Could you check a few things on this drawing? It's one solid part, dimensions in mm from its lowest x, y, z. A direction names the side the tool comes from. Give positions to 0.01 mm unless a question says otherwise; leave off trailing zeros. Order: outer loops, then holes, each group sorted by start corner. A loop starts at its lowest first (then second) coordinate and runs counter-clockwise, first axis right, second up. Notation, with made-up numbers: M -28.75,8 L -7.75,8 A19 cw -7.75,27 Z; hole C 53,3 d4. An arc over 180 degrees is marked long. Use one line per item in the form item = value.
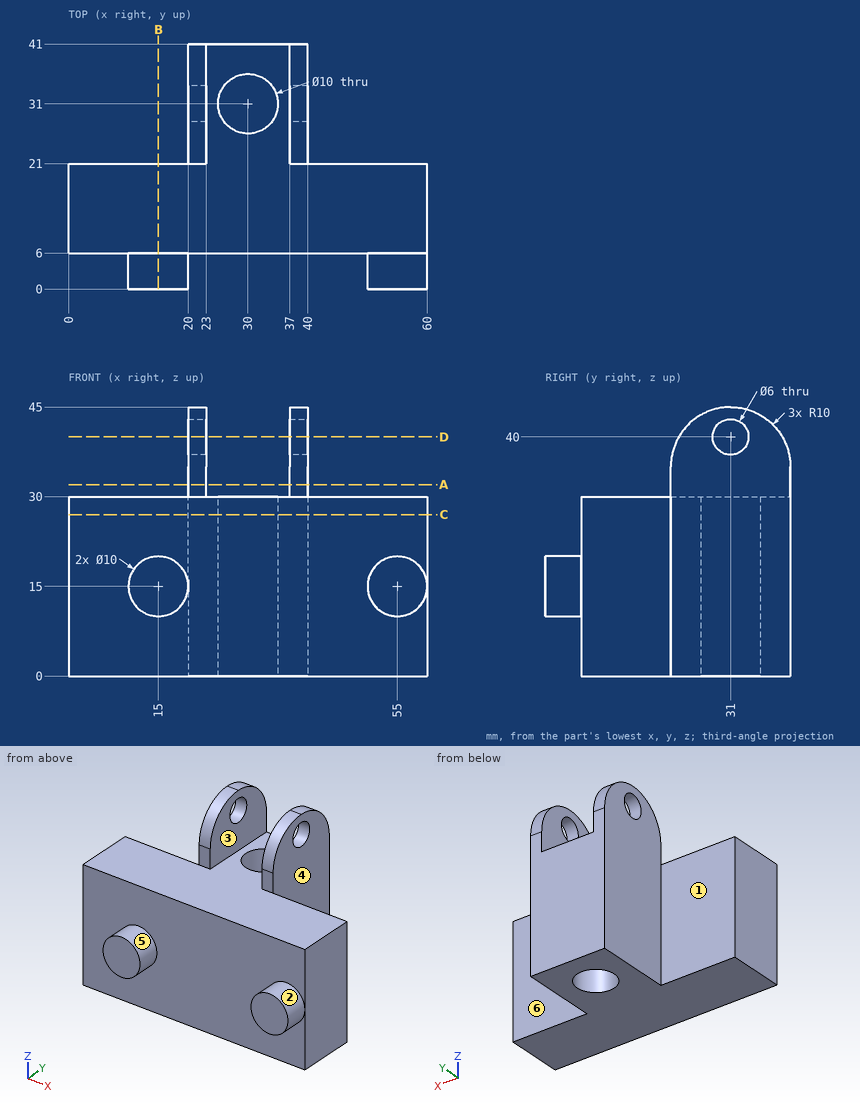
Q1. I want a section at D-D on z = 40. Write out the boundary of the cut face in (x, y), then the cut area to 3 significant figures.
Found:
outline = M 20,22.34 L 23,22.34 L 23,28 L 20,28 Z; M 20,34 L 23,34 L 23,39.66 L 20,39.66 Z; M 37,22.34 L 40,22.34 L 40,28 L 37,28 Z; M 37,34 L 40,34 L 40,39.66 L 37,39.66 Z
area = 67.9 mm²
Q2. I want a section at A-A on z = 32. Write out the boundary of the cut face in (x, y).
Found:
outline = M 20,21 L 23,21 L 23,41 L 20,41 Z; M 37,21 L 40,21 L 40,41 L 37,41 Z
Q3. I want a section at C-C on z = 27. Write out the boundary of the cut face in (x, y).
Found:
outline = M 0,6 L 60,6 L 60,21 L 40,21 L 40,41 L 20,41 L 20,21 L 0,21 Z; hole C 30,31 d10
Q4. I need wall thicknesses on L1, parallel to X at y = 27, z = 36; L2, parallel to X at y = 39, z = 4; L3, parallel to Z at x = 51, y = 8.5. Which ranges of each line are inside material? Lowest first, please.
Found:
L1 = 20 to 23, 37 to 40
L2 = 20 to 40
L3 = 0 to 30
Q5. I'm going to push flat-ended pins straight in: pin 1 Ø8 at (x, y) = (43, 10.5) entering from -Z; pin 2 Ø12 at (y, z) = (34, 39) entering from +X; pin 3 Ø8 at (x, z) = (24.5, 8.5) entering from -Y; pin 4 Ø10 at (x, z) = (49.5, 19.5) entering from +Y. Where does each tip first touch, or does it pass through?
Found:
pin_1 = 0
pin_2 = 40
pin_3 = 6
pin_4 = 21
Q6. Thinking about a two-plate mould opening in X: for the marked faces 4, 5 and 6, which applies, +X half, -X half, draft (parallel to the pull), parting line (faces both ways), or undercut?
Found:
face_4 = +X half
face_5 = undercut
face_6 = draft
Q7. I want a section at B-B on x = 15. Write out the boundary of the cut face in (y, z).
Found:
outline = M 0,10 L 6,10 L 6,0 L 21,0 L 21,30 L 6,30 L 6,20 L 0,20 Z
Q8. On a 3-axis mill with a long thin cutter (end or side, diameter ignored), from which of +Z, -Z, +X, -X, +Y, -Y can I reach the whole of each face in a straight line? I mean the marked faces 1, 2 and 3. Say none if no direction works.
Found:
face_1 = +Z, -Z, -X, +Y
face_2 = -Y
face_3 = +Z, +Y, -Y
